Geometry check sheet. Reference: drawing and pictorial views, mm from the part's lowest x, y, z. A direction names the side the tool comes from. Round coordinates to 2 decimals unless told otherwise and drop trailing zeros. Write each loop counter-clockwise with the first axis right and the second up, starting at its lowest first coordinate (ties: lowest second). Pieces come first, ordered by that corner, then holes. Notation, with made-up numbers: (55.25, -13.75) - (79.25, -13.75) arc R35 cw to (79.25, 20.25) - close; hole circle Ø11 at (25.25, -12). An arc over 180 degrees is marked (long way). Return JSON: item names as keys, results as strings.
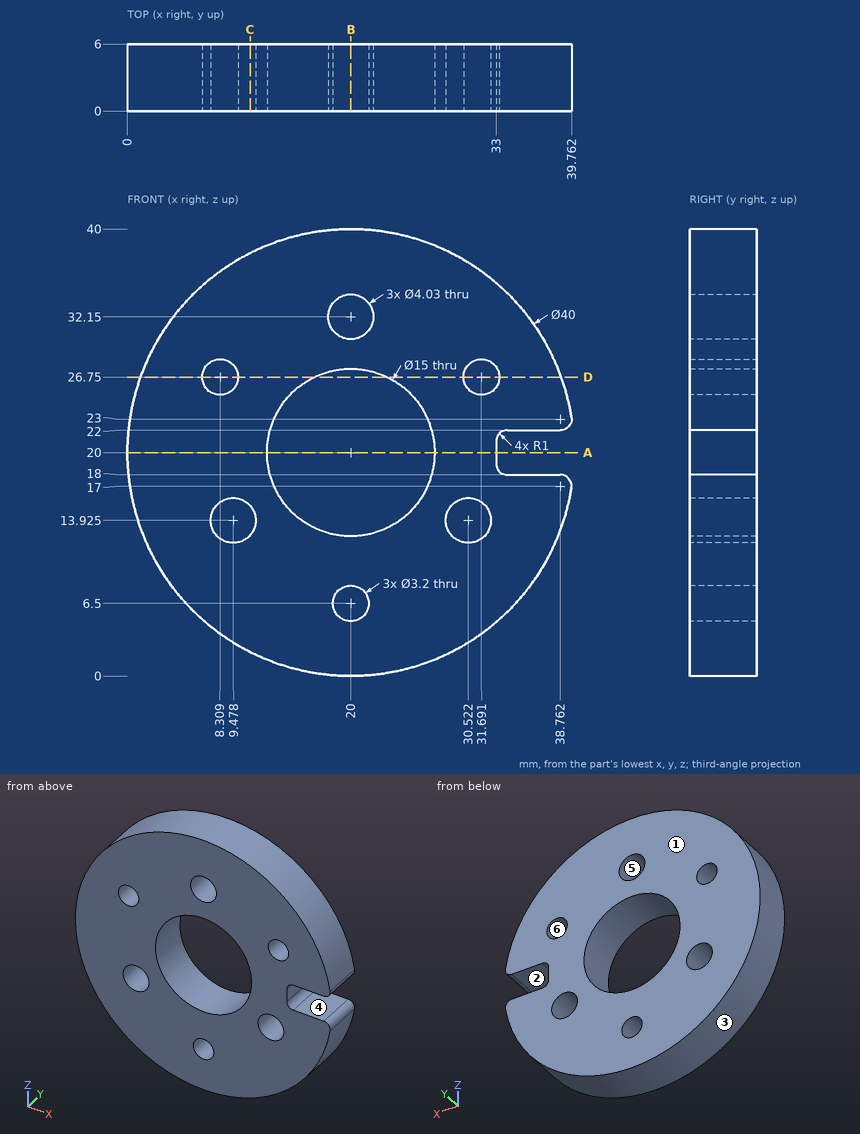
(1) Gauge pin test, flat ends, axial feed: pin 1 (1 mm diameter, centred on x = 25, y = 3, fed in from -Z); pin 2 (2.5 mm diameter, centred on x = 36, y = 3, fed in from -Z); pin 3 (3 mm diameter, centred on y = 4.5, z = 32.5, fed in from +X). Record the tip position at first contact, or that the pin passes through.
Response values:
{"pin 1": "stops at z = 0.51", "pin 2": "stops at z = 6.49", "pin 3": "stops at x = 36.7"}
(2) Section check A-A, the plane z = 20. Enter the section's corners in (x, y).
Response values:
{"outline": "(0, 0) - (12.5, 0) - (12.5, 6) - (0, 6) - close; (27.5, 0) - (33, 0) - (33, 6) - (27.5, 6) - close"}
(3) Section check B-B, the plane x = 20. Enter the section's corners in (y, z) (1 decimal), plus the area to 3 significant figures.
Response values:
{"outline": "(0, 0) - (6, 0) - (6, 4.9) - (0, 4.9) - close; (0, 8.1) - (6, 8.1) - (6, 12.5) - (0, 12.5) - close; (0, 27.5) - (6, 27.5) - (6, 30.1) - (0, 30.1) - close; (0, 34.2) - (6, 34.2) - (6, 40) - (0, 40) - close", "area": "107 mm^2"}
(4) Release check for a two-part mould opening along X. For the marked faces 3, 4, 5 and 6 record: pulls with the +X half, pulls with the -X half, needs draft (parallel to the pull), parting line crosses it, or undercut.
Response values:
{"face 3": "parting line crosses it", "face 4": "needs draft", "face 5": "undercut", "face 6": "undercut"}
(5) Section check C-C, the plane x = 11. Enter the section's corners in (y, z) (1 decimal).
Response values:
{"outline": "(0, 2.1) - (6, 2.1) - (6, 12.6) - (0, 12.6) - close; (0, 15.2) - (6, 15.2) - (6, 37.9) - (0, 37.9) - close"}
(6) Section check D-D, the plane z = 26.75. Enter the section's corners in (x, y), plus the area to 3 significant figures.
Response values:
{"outline": "(1.17, 0) - (6.71, 0) - (6.71, 6) - (1.17, 6) - close; (9.91, 0) - (16.73, 0) - (16.73, 6) - (9.91, 6) - close; (23.27, 0) - (30.09, 0) - (30.09, 6) - (23.27, 6) - close; (33.29, 0) - (38.83, 0) - (38.83, 6) - (33.29, 6) - close", "area": "148 mm^2"}
(7) Material ranges on line 1 along X through (y, z) = (0.5, 14) (1 decimal); line 2 along X through (y, z) = (4.1, 14.5) (1 decimal); line 3 along Z through (x, y) = (11, 4.85) (1 decimal), recorded low to high. Write a range as [from, to].
Response values:
{"line 1": "x = [0.9, 7.5], [11.5, 15.5], [24.5, 28.5], [32.5, 39.1]", "line 2": "x = [0.8, 7.5], [11.4, 14.9], [25.1, 28.6], [32.5, 39.2]", "line 3": "z = [2.1, 12.6], [15.2, 37.9]"}
(8) Access from +Z, -Z, +X, -X, +Y, -Y to the whole of each face (thin tool, end or side, straight path). Record for the marked faces 1 and 2.
Response values:
{"face 1": "+Z, -Z, +X, -X, +Y", "face 2": "+X, +Y, -Y"}
